CAD build for the part. Positions are in the model's coordinates, mm. Give positions to 0.01 mm unless a question says otherwise; leave off trailing zeros. Loops run counter-clockwise (first coordinate to the right, second up) from the corner with the lowest first, then second, coordinate; pieces in that order, holes last. Notation, with made-up numbers: (36, -16) -> (72, -16) arc R21 ccw to (72, -11) -> close; hole circle Ø6 at (-22, -21.5). An arc over 180 degrees is marked (long way). Write each question's results on one line, items separated by ' | '. Start each with the question number.
Autodesk Inventor part; units mm, degrees
ref_plane "YZ Plane" through (0, 0, 0) normal (1, 0, 0) x (0, 1, 0)
ref_plane "XZ Plane" through (0, 0, 0) normal (0, 1, 0) x (-1, 0, 0)
ref_plane "XY Plane" through (0, 0, 0) normal (0, 0, 1) x (1, 0, 0)
ref_plane "Work Plane1" through (0, 0, 5) normal (0, 0, 1) x (1, 0, 0)
sketch "Sketch1" plane through (0, 0, 5) normal (0, 0, 1) x (1, 0, 0)
  circle A0 centre (-39.5, 0) radius 1.5
  arc A1 (-39.5, 3) -> (-39.5, -3) centre (-39.5, 0) ccw
  line L0 (-39.5, -3) -> (-35.8748, -3)
  line L1 (-39.5, 3) -> (-35.8748, 3)
  circle A2 centre (39.5, 0) radius 1.5
  arc A3 (39.5, -3) -> (39.5, 3) centre (39.5, 0) ccw
  line L2 (39.5, -3) -> (35.8748, -3)
  line L3 (39.5, 3) -> (35.8748, 3)
  arc A4 (-35.8748, -3) -> (35.8748, -3) centre (0, 0) ccw
  arc A5 (35.8748, 3) -> (-35.8748, 3) centre (0, 0) ccw
extrude "Extrusion3" add sketch "Sketch1" along normal blind 1
properties part number "frame4"
Q1. Wall check: L1, parallel to Y at x = -39.5, z = 5.5; L2, parallel to Y at x = -36.5, z = 5.45; L3, parallel to X at y = 11, z = 5.6. Give the ranges that are in metal, low to high.
Q2. Saw through at D-D, the plane y = -18. List the corners of the cut face in (x, z).
Q3. Saw through at C-C, the plane x = -15. List the corners of the cut face in (y, z).
Q4. Drop flat-ended pins along their axis: pin 1 (3.5 mm diameter, centred on x = -39.5, y = 0, fed in from -Z); pin 2 (2.5 mm diameter, centred on x = 39.5, y = 0, fed in from +Z). Give the stop position or say it passes through.
Q5. Saw through at B-B, the plane z = 5.7. List the corners of the cut face in (x, y), then the cut area to 3 significant figures.
Q6. Saw through at A-A, the plane y = 0. List the corners of the cut face in (x, z).
Q7. Mould opens along Y. For faces 1 (the face through (0.75, -35.992, 5.493)), 2 (the face through (-1, 1, 5)), 3 (the face through (-42.5, -0.1, 5.5)), 4 (the face through (38.3, 0.9, 5.5)) say: pulls with the +Y half, pulls with the -Y half, needs draft (parallel to the pull), parting line crosses it, or undercut.
Answer block:
1) L1: y = -3 to -1.5, 1.5 to 3 | L2: y = -3 to 3 | L3: x = -34.28 to 34.28
2) outline: (-31.18, 5) -> (31.18, 5) -> (31.18, 6) -> (-31.18, 6) -> close
3) outline: (-32.73, 5) -> (32.73, 5) -> (32.73, 6) -> (-32.73, 6) -> close
4) pin 1: stops at z = 5 | pin 2: passes through
5) outline: (-39.5, -3) -> (-35.87, -3) arc R36 ccw to (35.87, -3) -> (39.5, -3) arc R3 ccw to (39.5, 3) -> (35.87, 3) arc R36 ccw to (-35.87, 3) -> (-39.5, 3) arc R3 ccw to start; hole circle Ø3 at (-39.5, 0); hole circle Ø3 at (39.5, 0) | area: 4,130 mm2
6) outline: (-42.5, 5) -> (-41, 5) -> (-41, 6) -> (-42.5, 6) -> close; (-38, 5) -> (38, 5) -> (38, 6) -> (-38, 6) -> close; (41, 5) -> (42.5, 5) -> (42.5, 6) -> (41, 6) -> close
7) face 1: pulls with the -Y half | face 2: needs draft | face 3: parting line crosses it | face 4: undercut
